Verification items for the finished model (mm, model axes). A direction names the side the tool comes from. Give positions to 0.01 mm unless a question says otherwise; leave off trailing zeros. Write each loop counter-clockwise with the first axis right and the second up, starting at its lowest first coordinate (ties: lowest second). Pieces come first, ordered by that corner, then holes. Notation, with made-up numbers: (-18.5, -13.75) -> (9.5, -13.75) arc R36 ccw to (9.5, 25.25) -> close; hole circle Ø6 at (-33, 53.5). An arc over 180 degrees is marked (long way). Answer as CSV lines item,"result". Start each with the question number.
1) Sectioned sample at D-D on z = 8.5. Record the cut outline in (x, y) (1 decimal).
2) Sectioned sample at B-B on x = 0. Record the cut outline in (y, z), and give its area (3 significant figures).
3) Mould release check, pull along Z, two halves, no side actions. Record for faces 3 (the cylindrical face through (19.31, 3.3, 30.15)), 4 (the flat face through (-0.1, -18.2, 0)), 5 (the cylindrical face through (-15.921, 17.945, 50.089)): released by +Z, released by -Z, zero draft, split by the parting line, or undercut.
4) Sectioned sample at C-C on y = 11.5. Record the cut outline in (x, z), and give its area (3 significant figures).
5) Sectioned sample at A-A on y = 0. Record the cut outline in (x, z).
6) Material ranges on L1, parallel to Z at x = 0, y = -18.75; L2, parallel to X at y = 9, z = 55; L3, parallel to Y at x = -16, z = 73.5, recorded low to high.
7) Tool access check on faces 1 (the flat face through (17.945, -1, 50)), 2 (the cylindrical face through (-19.87, -19.83, 50.09)). Record the directions out of +Z, -Z, +X, -X, +Y, -Y that give a thin tool (end or side, any length) a straight path to the whole face; none if there is none.
8) Gauge pin test, flat ends, axial feed: pin 1 Ø16.5 at (y, z) = (0, 23.81) entering from -X; pin 2 Ø8.5 at (x, z) = (0, 71.44) entering from +Y. Record the tip position at first contact, or that the pin passes through.
```python
from build123d import *

# Parameters (mm, degrees)
BASE_EXTRUDE_DEPTH                        = 101.6
HOLE1_START                               = -20.6375
HOLE1_OUTLINE_R                           = 7.14375
HOLE1_DEPTH                               = 2.6924
LPATTERN1_COUNT                           = 2
LPATTERN1_PITCH                           = 47.625
CIRPATTERN1_COUNT                         = 2
CIRPATTERN1_ANGLE                         = 90
CIRPATTERN1_START                         = -20.6375
CIRPATTERN1_COPY_1_SKETCH_R               = 7.14375
CIRPATTERN1_COPY_1_DEPTH                  = 2.6924
CIRPATTERN1_THE_OTHER_WAY_COUNT           = 2
CIRPATTERN1_THE_OTHER_WAY_ANGLE           = 90
CIRPATTERN1_THE_OTHER_WAY_COPY_1_SKETCH_R = 7.14375
CIRPATTERN1_THE_OTHER_WAY_COPY_1_DEPTH    = 2.6924


# Read off the part's stored shape, not the designer's step: Hole1
with BuildPart() as part:
    # Sketch1 → Base-Extrude (new body)
    with BuildSketch(Plane.XY):
        with BuildLine():
            Line((-20.6375, 15.875), (-20.6375, -17.9451))
            ThreePointArc((-20.6375, -17.9451), (-19.848914298, -19.848914298), (-17.9451, -20.6375))
            Line((-17.9451, -20.6375), (17.9451, -20.6375))
            ThreePointArc((17.9451, -20.6375), (19.848914298, -19.848914298), (20.6375, -17.9451))
            Line((20.6375, -17.9451), (20.6375, 15.875))
            ThreePointArc((20.6375, 15.875), (15.875, 20.6375), (11.1125, 15.875))
            Line((11.1125, 15.875), (11.1125, 14.83995))
            ThreePointArc((11.1125, 14.83995), (12.4587, 13.49375), (13.8049, 14.83995))
            Line((13.8049, 14.83995), (13.8049, 15.875))
            ThreePointArc((13.8049, 15.875), (15.875, 17.9451), (17.9451, 15.875))
            Line((17.9451, 15.875), (17.9451, -17.9451))
            Line((17.9451, -17.9451), (-17.9451, -17.9451))
            Line((-17.9451, -17.9451), (-17.9451, 15.875))
            ThreePointArc((-17.9451, 15.875), (-15.875, 17.9451), (-13.8049, 15.875))
            Line((-13.8049, 15.875), (-13.8049, 14.83995))
            ThreePointArc((-13.8049, 14.83995), (-12.4587, 13.49375), (-11.1125, 14.83995))
            Line((-11.1125, 14.83995), (-11.1125, 15.875))
            ThreePointArc((-11.1125, 15.875), (-15.875, 20.6375), (-20.6375, 15.875))
        make_face()
    extrude(amount=BASE_EXTRUDE_DEPTH)

    # Hole1 outline → Hole1 (cut)
    with BuildSketch(Plane(origin=(0, 0, 0), x_dir=(1, 0, 0), z_dir=(0, 1, 0)).offset(HOLE1_START)):
        with Locations((0, -23.8125)):
            Circle(HOLE1_OUTLINE_R)
    hole1 = extrude(amount=HOLE1_DEPTH, mode=Mode.SUBTRACT)

    # LPattern1: Hole1 ×2
    with Locations(*[(0, 0, i * LPATTERN1_PITCH) for i in range(1, LPATTERN1_COUNT)]):
        add(hole1, mode=Mode.SUBTRACT)

    # CirPattern1: Hole1 ×2 about axis
    cirpattern1_axis = Axis((0, 0, -50), (0, 0, 1))
    for i in range(1, CIRPATTERN1_COUNT):
        add(hole1.rotate(cirpattern1_axis, i * CIRPATTERN1_ANGLE / (CIRPATTERN1_COUNT - 1)), mode=Mode.SUBTRACT)

    # CirPattern1 copy 1 sketch → CirPattern1 copy 1 (cut)
    with BuildSketch(Plane(origin=(0, 0, 47.625), x_dir=(0, 1, 0), z_dir=(-1, 0, 0)).offset(CIRPATTERN1_START)):
        with Locations((0, -23.8125)):
            Circle(CIRPATTERN1_COPY_1_SKETCH_R)
    extrude(amount=CIRPATTERN1_COPY_1_DEPTH, mode=Mode.SUBTRACT)

    # CirPattern1 the other way: Hole1 ×2 about axis
    cirpattern1_the_other_way_axis = Axis((0, 0, -50), (0, 0, -1))
    for i in range(1, CIRPATTERN1_THE_OTHER_WAY_COUNT):
        add(hole1.rotate(cirpattern1_the_other_way_axis, i * CIRPATTERN1_THE_OTHER_WAY_ANGLE / (CIRPATTERN1_THE_OTHER_WAY_COUNT - 1)), mode=Mode.SUBTRACT)

    # CirPattern1 the other way copy 1 sketch → CirPattern1 the other way copy 1 (cut)
    with BuildSketch(Plane(origin=(0, 0, 47.625), x_dir=(0, -1, 0), z_dir=(1, 0, 0)).offset(CIRPATTERN1_START)):
        with Locations((0, -23.8125)):
            Circle(CIRPATTERN1_THE_OTHER_WAY_COPY_1_SKETCH_R)
    extrude(amount=CIRPATTERN1_THE_OTHER_WAY_COPY_1_DEPTH, mode=Mode.SUBTRACT)


solid = part.part
```
Ans:
1,outline,"(-20.6, -17.9) arc R2.7 ccw to (-17.9, -20.6) -> (17.9, -20.6) arc R2.7 ccw to (20.6, -17.9) -> (20.6, 15.9) arc R4.8 ccw to (11.1, 15.9) -> (11.1, 14.8) arc R1.3 ccw to (13.8, 14.8) -> (13.8, 15.9) arc R2.1 cw to (17.9, 15.9) -> (17.9, -17.9) -> (-17.9, -17.9) -> (-17.9, 15.9) arc R2.1 cw to (-13.8, 15.9) -> (-13.8, 14.8) arc R1.3 ccw to (-11.1, 14.8) -> (-11.1, 15.9) arc R4.8 ccw to (-20.6, 15.9) -> close"
2,outline,"(-20.64, 0) -> (-17.95, 0) -> (-17.95, 16.67) -> (-20.64, 16.67) -> close; (-20.64, 30.96) -> (-17.95, 30.96) -> (-17.95, 64.29) -> (-20.64, 64.29) -> close; (-20.64, 78.58) -> (-17.95, 78.58) -> (-17.95, 101.6) -> (-20.64, 101.6) -> close"
2,area,"197 mm²"
3,face 3,"undercut"
3,face 4,"released by -Z"
3,face 5,"zero draft"
4,outline,"(-20.64, 0) -> (-17.95, 0) -> (-17.95, 101.6) -> (-20.64, 101.6) -> close; (17.95, 0) -> (20.64, 0) -> (20.64, 101.6) -> (17.95, 101.6) -> close"
4,area,"547 mm²"
5,outline,"(-20.64, 0) -> (-17.95, 0) -> (-17.95, 16.67) -> (-20.64, 16.67) -> close; (-20.64, 30.96) -> (-17.95, 30.96) -> (-17.95, 64.29) -> (-20.64, 64.29) -> close; (-20.64, 78.58) -> (-17.95, 78.58) -> (-17.95, 101.6) -> (-20.64, 101.6) -> close; (17.95, 0) -> (20.64, 0) -> (20.64, 16.67) -> (17.95, 16.67) -> close; (17.95, 30.96) -> (20.64, 30.96) -> (20.64, 64.29) -> (17.95, 64.29) -> close; (17.95, 78.58) -> (20.64, 78.58) -> (20.64, 101.6) -> (17.95, 101.6) -> close"
6,L1,"z = 0 to 16.67, 30.96 to 64.29, 78.58 to 101.6"
6,L2,"x = -20.64 to -17.95, 17.95 to 20.64"
6,L3,"y = -20.64 to -17.95, 17.94 to 20.64"
7,face 1,"+Z, -Z"
7,face 2,"+Z, -Z, -X, -Y"
8,pin 1,"stops at x = -20.64"
8,pin 2,"passes through"
